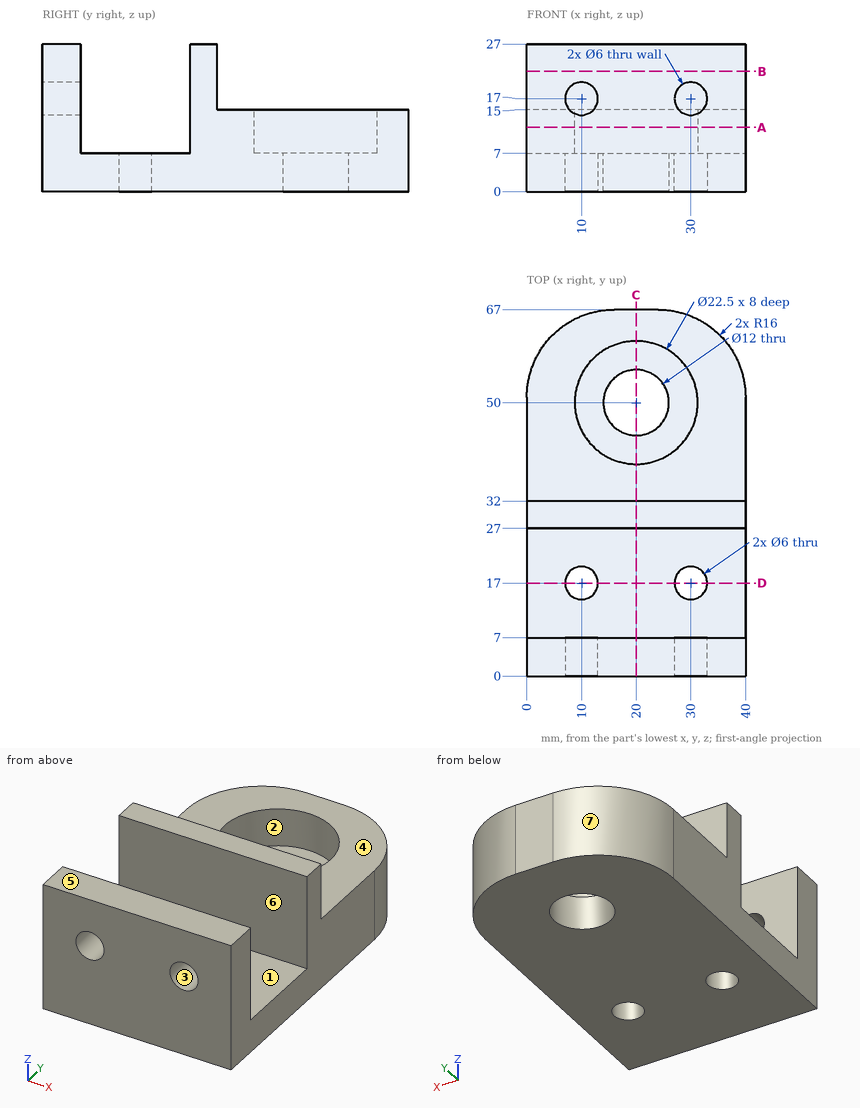
Could you check a few things on this drawing? It's one solid part, dimensions in mm from its lowest x, y, z. A direction names the side the tool comes from. Coordinates: 2 decimals unless noted, no trailing zeros. Order: outer loops, then holes, each group sorted by start corner. A loop starts at its lowest first (then second) coordinate and runs counter-clockwise, first axis right, second up. Notation, with made-up numbers: (18.25, -35) - (65.25, -35) arc R14 cw to (65.25, -13) - close; hole circle Ø11 at (48.25, 12.25). An arc over 180 degrees is marked (long way). Answer as a JSON object with one key per item and string values. Group by question number.
Q1. Imagine slicing it at A-A (z = 11.75). Please give me the cut outline in (x, y).
Q2. On a 3-axis mill with a long thin cutter (end or side, diameter ignored), from which of +Z, -Z, +X, -X, +Y, -Y can I reach the whole of each face in a straight line? I mean the marked faces 1, 2, 3 and 4. Say none if no direction works.
Q3. Imagine slicing it at D-D (y = 17). Please give me the cut outline in (x, z), and give its area (3 significant figures).
Q4. We'd pull the mould along Y, two halves only. Please class the marked faces 5, 6 and 7: +Y half, -Y half, draft (parallel to the pull), parting line (faces both ways), or undercut.
Q5. I need wall thicknesses on line 1 (Y direction, x = 20, z = 10); line 2 (Y direction, x = 32.5, z = 19.5); line 3 (Z direction, x = 30, y = 2.25). Which ranges of each line are inside material? Lowest first, please. Write a range as from..to.
Q6. Will these pins go through, and if not, where does the flat tip stop? P1, Ø13, axis at x = 25.5, z = 23, coming from the +Y side; P2, Ø8, axis at x = 30, z = 17, coming from the +Y side; P3, Ø20, axis at x = 20, y = 50, coming from the +Z side.
Q7. Imagine slicing it at C-C (x = 20). Please give me the cut outline in (y, z).
Q8. Imagine slicing it at B-B (z = 22). Please give me the cut outline in (x, y).
Determined:
{
 "1": {"outline": "(0, 0) - (40, 0) - (40, 7) - (0, 7) - close; (0, 27) - (40, 27) - (40, 51) arc R16 ccw to (24, 67) - (16, 67) arc R16 ccw to (0, 51) - close; hole circle Ø22.5 at (20, 50)"},
 "2": {"face 1": "+Z, +X, -X", "face 2": "+Z", "face 3": "-Y", "face 4": "+Z, +X, -X, +Y"},
 "3": {"outline": "(0, 0) - (7, 0) - (7, 7) - (0, 7) - close; (13, 0) - (27, 0) - (27, 7) - (13, 7) - close; (33, 0) - (40, 0) - (40, 7) - (33, 7) - close", "area": "196 mm2"},
 "4": {"face 5": "draft", "face 6": "undercut", "face 7": "+Y half"},
 "5": {"line 1": "y = 0..7, 27..38.75, 61.25..67", "line 2": "y = 0..7, 27..32", "line 3": "z = 0..14, 20..27"},
 "6": {"P1": "stops at y = 32", "P2": "stops at y = 66.8", "P3": "stops at z = 7"},
 "7": {"outline": "(0, 0) - (44, 0) - (44, 7) - (38.75, 7) - (38.75, 15) - (32, 15) - (32, 27) - (27, 27) - (27, 7) - (7, 7) - (7, 27) - (0, 27) - close; (56, 0) - (67, 0) - (67, 15) - (61.25, 15) - (61.25, 7) - (56, 7) - close"},
 "8": {"outline": "(0, 0) - (40, 0) - (40, 7) - (0, 7) - close; (0, 27) - (40, 27) - (40, 32) - (0, 32) - close"}
}
